Here's how the part is built. I have some questions about the finished solid (model axes, mm). Face numbers are marked on the shaded views. Round coordinates to 2 decimals unless told otherwise and drop trailing zeros. Loops run counter-clockwise (first coordinate to the right, second up) from the corner with the lowest first, then second, coordinate; pieces in that order, holes last. Notation, with made-up numbers: M -6.5,-11.5 L 37.5,-11.5 A20 cw 37.5,3.5 Z; hole C 38,-35 d4. An arc over 180 degrees is marked long. Answer as CSV lines item,"result".
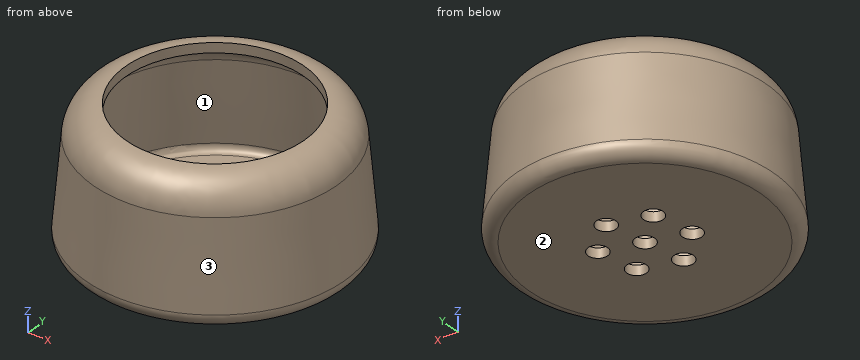
```python
from build123d import *

# Parameters (mm, degrees)
F0_R     = 50.8
F1_DEPTH = 50.8
F1_TAPER = 5
F2_R     = 12.7
F3_T     = -3.81
F4_R     = 2.54
F6_D     = 7.62
F7_R     = 5.08


# Not quite as in the source:
# - a shell that OpenCascade refuses in one call is made with other operations: the cavity is built on its own and cut out


with BuildPart() as f1:
    # F0 (on Top) → F1 (new body)
    with BuildSketch(Plane.XY):
        Circle(F0_R)
    extrude(amount=F1_DEPTH, taper=F1_TAPER)

    # F2
    f2_edges = [f1.edges().sort_by_distance(p)[0] for p in [
        (-46.355576, 0, 50.8),
    ]]
    fillet(f2_edges, radius=F2_R)

    # F3: a shell. OpenCascade refuses it in one call, so the cavity is built on its own and cut out:
    # the body offset inwards by the wall thickness, plus a prism from it out through each open face.
    f3_core = offset(f1.part, amount=F3_T, mode=Mode.PRIVATE)
    f3_exits = [f3_core.faces().sort_by_distance(p)[0] for p in [
        (0, 0, 46.99),
    ]]
    add(f3_core, mode=Mode.SUBTRACT)
    extrude(f3_exits, amount=-F3_T, mode=Mode.SUBTRACT)

    # F4
    f4_edges = [f1.edges().sort_by_distance(p)[0] for p in [
        (-46.642115, 0, 3.81),
    ]]
    fillet(f4_edges, radius=F4_R)

    # F6 (through all)
    with Locations(Plane(origin=(0, 0, 0), x_dir=(1, 0, 0), z_dir=(0, 0, -1))):
        with Locations((3.3266340716, -15.1329960019), (-11.4422419373, -10.4474476161), (-14.7688760089, 4.6855483859), (-3.3266340716, 15.1329960019), (11.4422419373, 10.4474476161), (14.7688760089, -4.6855483859), (0, 0)):
            Hole(F6_D / 2)

    # F7
    f7_edges = [f1.edges().sort_by_distance(p)[0] for p in [
        (-50.8, 0, 0),
    ]]
    fillet(f7_edges, radius=F7_R)


solid = f1.part
```
1. If I drill on line 1 (Y direction, x = 0, z = 1); line 2 (Z direction, x = -28.5, y = -0.5); line 3 (Y direction, x = -32.5, z = 32.5), over which ranges is the centre line in solid material (lowest first)? Write a range as [from, to].
Evaluation:
line 1,"y = [-48.28, -16.99], [-13.28, -3.81], [3.81, 13.28], [16.99, 48.28]"
line 2,"z = [0, 3.81]"
line 3,"y = [-35.26, -29.86], [29.86, 35.26]"
2. We'd pull the mould along Z, two halves only. Please class the marked faces 1, 2 and 3: pulls with the +Z half, pulls with the -Z half, needs draft (parallel to the pull), parting line crosses it, or undercut.
Evaluation:
face 1,"undercut"
face 2,"pulls with the -Z half"
face 3,"pulls with the +Z half"
3. For P1, Ø1.5, axis at x = 22.5, z = 43.5, coming from the -Y side; P2, Ø5, axis at x = 19.5, z = 40, coming from the +Y side; P3, Ø8, axis at y = 26.5, z = 10.5, coming from the +X side, each with a flat end and sliding along its axis, tell me the tip position at first contact or that it passes through.
Evaluation:
P1,"stops at y = -40.92"
P2,"stops at y = 44.17"
P3,"stops at x = 44.56"
4. I want a section at A-A, the plane z = 43. Please give me the cut outline in (x, y), and give its area (3 significant figures).
Evaluation:
outline,"C 0,0 d92.87; hole C 0,0 d84.27"
area,"1,200 mm²"
5. I want a section at B-B, the plane z = 34. Please give me the cut outline in (x, y), and give its area (3 significant figures).
Evaluation:
outline,"C 0,0 d95.65; hole C 0,0 d88"
area,"1,100 mm²"
